Part model, mm, in its own coordinate system. A direction names the side the tool comes from. Give positions to 0.01 mm unless a question says otherwise; leave off trailing zeros. Order: outer loops, then holes, each group sorted by start corner. A loop starts at its lowest first (then second) coordinate and runs counter-clockwise, first axis right, second up. Notation, with made-up numbers: M 30.25,-18 L 79.25,-18 A24 cw 79.25,19 Z; hole C -27.5,71 d10. An arc over 180 degrees is marked long. Answer as a JSON object with one key per item and string values.
from build123d import *

# Parameters (mm, degrees)
SKETCH036_R             = 2.75
PAD021_DEPTH            = 3
SKETCH037_R             = 1.5
PAD022_DEPTH            = 6
POCKET017_DEPTH         = 4
BODY010_PLACEMENT_ANGLE = 225


with BuildPart() as part:
    # Sketch036 → Pad021 (new body)
    with BuildSketch(Plane.XY):
        Circle(SKETCH036_R)
    extrude(amount=PAD021_DEPTH)

    # Sketch037 (on Face2 of Pad021) → Pad022 (join)
    with BuildSketch(Plane(origin=(0, 0, 0), x_dir=(1, 0, 0), z_dir=(0, 0, -1))):
        Circle(SKETCH037_R)
    extrude(amount=PAD022_DEPTH)

    # Sketch038 (on DatumPlane) → Pocket017 (cut)
    with BuildSketch(Plane.XY.offset(3)):
        Polygon((0.721688, -1.25), (1.443376, 0), (0.721688, 1.25), (-0.721688, 1.25), (-1.443376, 0), (-0.721688, -1.25), align=None)
    extrude(amount=-POCKET017_DEPTH, mode=Mode.SUBTRACT)


with BuildPart() as part_1:
    # Body010 placement: moved
    add(part.part.moved(Location((-118.5, -61.871843, 6.010408))).rotate(Axis((-118.5, -61.871843, 6.010408), (1, 0, 0)), BODY010_PLACEMENT_ANGLE))


solid = part_1.part
1. Cut at A-A on x = -118.15. Give the cut face in (y, z), plus the area to 3 significant figures.
Worked answers:
{"outline": "M -67.15,9.22 L -62.9,4.98 L -63.8,4.08 L -61.68,1.96 L -60.63,3.01 L -63.46,5.83 L -61.7,7.6 L -58.87,4.77 L -57.82,5.82 L -59.94,7.94 L -60.84,7.04 L -65.08,11.28 Z", "area": "23.9 mm^2"}
2. Cut at C-C on x = -120.7. Give the cut face in (y, z), plus the area to 3 significant figures.
Worked answers:
{"outline": "M -63.04,4.84 L -60.92,2.72 L -58.58,5.06 L -60.71,7.18 Z", "area": "9.90 mm^2"}
3. Two-plate mould, pull along X, no slides. Class faces 3 (the cylindrical face through (-120, -63.9, 8.1)), 4 (the flat face through (-119.588, -60.709, 5.719)), 5 (the flat face through (-117.32, -61.03, 6.85)): +X half, -X half, draft (parallel to the pull), parting line (faces both ways), or undercut.
Worked answers:
{"face 3": "parting line", "face 4": "undercut", "face 5": "draft"}
4. Probe line 1 along X through (y, z) = (-63, 6.25); line 2 along X through (y, z) = (-61.5, 7.25); line 3 along Z through (x, y) = (-118.3, -60.75). List the from-to ranges inside material, lowest first.
Worked answers:
{"line 1": "x = -119.86 to -119.58, -117.42 to -117.14", "line 2": "x = -119.48 to -119.29, -117.71 to -117.52", "line 3": "z = 2.89 to 3.12, 6.66 to 7.13"}
5. Which spindle directions (+Z, -Z, +X, -X, +Y, -Y) get a long thin tool onto all of the face, cutting with end or side? Do faces 1 (the flat face through (-118.52, -66.1, 10.27)), 2 (the flat face through (-117.41, -61.58, 4.85)). Say none if no direction does.
Worked answers:
{"face 1": "+Z, +X, -X, -Y", "face 2": "none"}
6. Pin check, flat tip, straight feed: P1, Ø1, axis at y = -59.5, z = 6, coming from the -X side. Stop position of the tip, or through.
Worked answers:
{"P1": "stops at x = -120.99"}
7. Cut at B-B on x = -116.5. Give the cut face in (y, z), plus the area to 3 significant figures.
Worked answers:
{"outline": "M -63.21,4.68 L -61.09,2.55 L -58.42,5.22 L -60.54,7.35 Z", "area": "11.3 mm^2"}
